Can you work these out from the model? Positions are in its coordinate system, mm. Coordinates: 2 decimals unless noted, no trailing zeros. Order: outer loops, then holes, each group sorted by start corner. A loop starts at its lowest first (then second) coordinate and runs counter-clockwise, first axis right, second up. Notation, with made-up numbers: (79.25, 20) -> (114.25, 20) arc R9 cw to (114.25, 36) -> close; hole circle Ø2 at (59, -23.5). An arc over 180 degrees is marked (long way). Return JSON: item names as keys, results as strings. Group by question number.
1) If I drill on probe 1 along Y at (x, z) = (0, 2.15) (3 decimals); probe 2 along X at (y, z) = (-2, 3); probe 3 along Y at (x, z) = (-19.5, 1.1), over which ranges is the centre line in solid material (lowest first)? Write a range as from..to.
2) For pin 1 (1 mm diameter, centred on y = -10.5, z = 2, fed in from -X); pin 2 (1.5 mm diameter, centred on x = -23, z = 0.5, fed in from -Y); pin 3 (3 mm diameter, centred on x = 49.49, y = -28.58, fed in from -Z); pin 4 (1 mm diameter, centred on x = -10, z = 0.5, fed in from -Y), each with a flat end and sliding along its axis, tell me the tip position at first contact or that it passes through.
3) If we section it at B-B, the plane x = 17: Please give me the cut outline in (y, z) (3 decimals), then the cut area to 3 significant figures.
4) If we section it at A-A, the plane y = 0: Please give me the cut outline in (x, z) (3 decimals).
5) If we section it at D-D, the plane z = 2.1: State how many separate pieces and enclosed holes the cut face has, then the cut area to 3 significant figures.
6) If we section it at C-C, the plane y = -63: Please give me the cut outline in (x, z) (3 decimals).
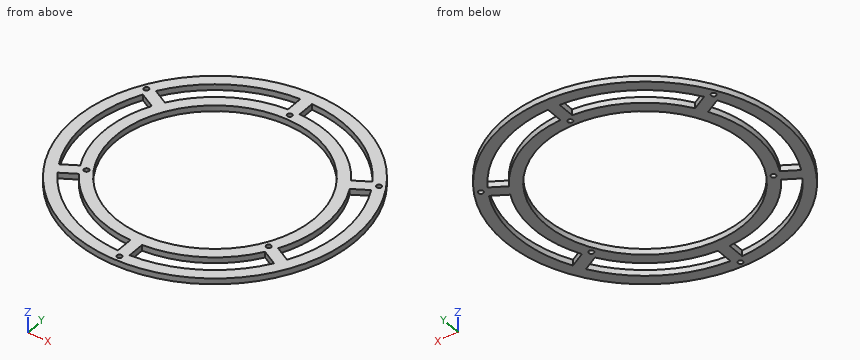
from build123d import *

# Parameters (mm, degrees)
F0_R            = 76.2
F0_R_2          = 1.35255
F0_R_3          = 53.975
F1_DEPTH        = 3.175
F3_DEPTH        = 3.175
F3_COPIES_COUNT = 6


# Not quite as in the source:
# - a pattern or mirror of a feature is missing from the dataset's text; its kind, count and spacing are read off the source's solid


with BuildPart() as f1:
    # F0 (on Top) → F1 (new body)
    with BuildSketch(Plane.XY):
        Circle(F0_R)
        with Locations((-49.4933518263, -28.575)):
            Circle(F0_R_2, mode=Mode.SUBTRACT)
        with Locations((0, -73.025)):
            Circle(F0_R_2, mode=Mode.SUBTRACT)
        with Locations((49.4933518263, -28.575)):
            Circle(F0_R_2, mode=Mode.SUBTRACT)
        with Locations((-63.2415051114, 36.5125)):
            Circle(F0_R_2, mode=Mode.SUBTRACT)
        Circle(F0_R_3, mode=Mode.SUBTRACT)
        with Locations((63.2415051114, 36.5125)):
            Circle(F0_R_2, mode=Mode.SUBTRACT)
        with Locations((0, 57.15)):
            Circle(F0_R_2, mode=Mode.SUBTRACT)
    extrude(amount=F1_DEPTH)

    # F2 (on face) → F3 (cut, through all)
    with BuildSketch(Plane.XY.offset(3.175)):
        with BuildLine():
            ThreePointArc((-53.7580736024, -27.3710640561), (-60.325, 0), (-53.7580736024, 27.3710640561))
            Line((-53.7580736024, 27.3710640561), (-62.0168505364, 32.1392711421))
            ThreePointArc((-62.0168505364, 32.1392711421), (-69.85, 0), (-62.0168505364, -32.1392711421))
            Line((-62.0168505364, -32.1392711421), (-53.7580736024, -27.3710640561))
        make_face()
    f3 = extrude(amount=-F3_DEPTH, mode=Mode.SUBTRACT)

    # F3_copies: F3 ×6 about axis
    f3_copies_axis = Axis((0, 0, 0), (0, 0, 1))
    for i in range(1, F3_COPIES_COUNT):
        add(f3.rotate(f3_copies_axis, i * 360 / F3_COPIES_COUNT), mode=Mode.SUBTRACT)


solid = f1.part
Result sheet:
{
 "1": {"probe 1": "y = -76.2..-74.378, -71.672..-53.975, 53.975..55.797, 58.503..76.2", "probe 2": "x = -76.17..-69.82, -60.29..-53.94, 53.94..60.29, 69.82..76.17", "probe 3": "y = -73.66..-67.07, -57.09..-50.33, 50.33..57.09, 67.07..73.66"},
 "2": {"pin 1": "stops at x = -75.54", "pin 2": "stops at y = -72.88", "pin 3": "stops at z = 0", "pin 4": "stops at y = -75.61"},
 "3": {"outline": "(-74.279, 0) -> (-67.75, 0) -> (-67.75, 3.175) -> (-74.279, 3.175) -> close; (-57.88, 0) -> (-51.228, 0) -> (-51.228, 3.175) -> (-57.88, 3.175) -> close; (51.228, 0) -> (57.88, 0) -> (57.88, 3.175) -> (51.228, 3.175) -> close; (67.75, 0) -> (74.279, 0) -> (74.279, 3.175) -> (67.75, 3.175) -> close", "area": "83.7 mm2"},
 "4": {"outline": "(-76.2, 0) -> (-69.85, 0) -> (-69.85, 3.175) -> (-76.2, 3.175) -> close; (-60.325, 0) -> (-53.975, 0) -> (-53.975, 3.175) -> (-60.325, 3.175) -> close; (53.975, 0) -> (60.325, 0) -> (60.325, 3.175) -> (53.975, 3.175) -> close; (69.85, 0) -> (76.2, 0) -> (76.2, 3.175) -> (69.85, 3.175) -> close"},
 "5": {"separate pieces": "1", "enclosed holes": "13", "area": "5,520 mm2"},
 "6": {"outline": "(-42.865, 0) -> (-30.167, 0) -> (-30.167, 3.175) -> (-42.865, 3.175) -> close; (-3.175, 0) -> (3.175, 0) -> (3.175, 3.175) -> (-3.175, 3.175) -> close; (30.167, 0) -> (42.865, 0) -> (42.865, 3.175) -> (30.167, 3.175) -> close"}
}
